```python
from build123d import *

# Parameters (mm, degrees)
F0_R     = 48.989285
F1_DEPTH = 99
F2_R     = 5
F3_R     = 5


with BuildPart() as f1:
    # F0 (on Top) → F1 (new body)
    with BuildSketch(Plane.XY):
        with Locations((90.133347, 19.112047)):
            Circle(F0_R)
    extrude(amount=F1_DEPTH)

    # F2
    f2_edges = [f1.edges().sort_by_distance(p)[0] for p in [
        (41.144062, 19.112047, 0),
    ]]
    fillet(f2_edges, radius=F2_R)

    # F3
    f3_edges = [f1.edges().sort_by_distance(p)[0] for p in [
        (41.144062, 19.112047, 99),
    ]]
    fillet(f3_edges, radius=F3_R)


solid = f1.part
```
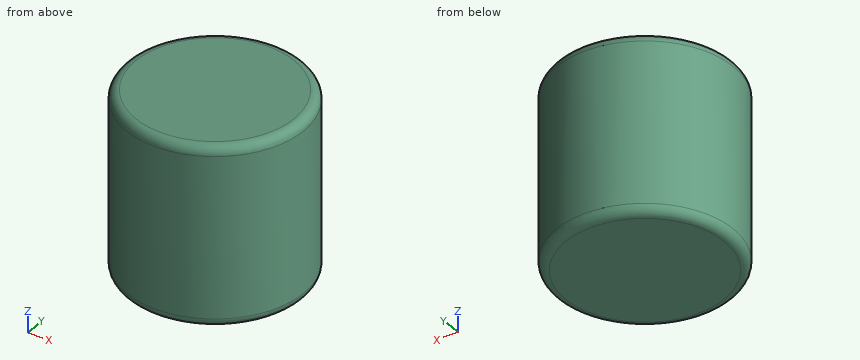
Verification items for the finished model (mm, model axes). Give positions to 0.01 mm unless a question says otherwise; leave off trailing zeros. Order: outer loops, then holes, each group sorted by start corner. A loop starts at its lowest first (then second) coordinate and runs counter-clockwise, first axis right, second up. Notation, with made-up numbers: M 69,-4.5 L 109,-4.5 A19 cw 109,21.5 Z; hole C 5.25,-5.75 d10. An arc over 180 degrees is marked long. Answer in a Markdown table with one row per item. Add a question column.
Item 1: Gauge pin test, flat ends, axial feed: pin 1 (6 mm diameter, centred on x = 105, z = 63, fed in from +Y); pin 2 (5 mm diameter, centred on x = 118.5, z = 50.5, fed in from +Y); pin 3 (3 mm diameter, centred on y = -6, z = 71, fed in from -X). Record the tip position at first contact, or that the pin passes through.
Item 2: Section check A-A, the plane z = 65.5. Enter the section's corners in (x, y), and give its area (3 significant figures).
Item 3: Scan lines: probe 1 along Z at (x, y) = (118, 55.5); probe 2 along X at (y, z) = (43, 17.5); probe 3 along X at (y, z) = (-20, 92). Record each from-to range of solid material in increasing order. Write a range as from..to.
Filled sheet:
| question | item | result |
|---|---|---|
| 1 | pin 1 | stops at y = 66.64 |
| 1 | pin 2 | stops at y = 60.72 |
| 1 | pin 3 | stops at x = 47.21 |
| 2 | outline | C 90.13,19.11 d97.98 |
| 2 | area | 7,540 mm^2 |
| 3 | probe 1 | z = 0.35..98.65 |
| 3 | probe 2 | x = 47.36..132.9 |
| 3 | probe 3 | x = 60.63..119.63 |
